Build history of the part. All positions in model axes, mm. A direction names the side the tool comes from. Coordinates: 2 decimals unless noted, no trailing zeros. Order: outer loops, then holes, each group sorted by start corner. A loop starts at its lowest first (then second) coordinate and runs counter-clockwise, first axis right, second up. Notation, with made-up numbers: M 7,62 L 28,62 A25 ccw 28,88 Z; hole C -17,85 d6. An arc over 180 degrees is marked long. Use a Markdown table: item, result. Add a question column.
from build123d import *

# Parameters (mm, degrees)
SKETCH1_W           = 124
SKETCH1_H           = 84
BOSS_EXTRUDE1_DEPTH = 25
SKETCH2_W           = 112
SKETCH2_H           = 73
CUT_EXTRUDE1_DEPTH  = 20
SKETCH4_W           = 2
SKETCH4_H           = 7
SKETCH4_H_2         = 36.5
CUT_EXTRUDE2_DEPTH  = 20
FILLET1_R           = 2.5
SKETCH5_W           = 119
SKETCH5_H           = 5
BOSS_EXTRUDE2_DEPTH = 10
SKETCH6_W           = 117
SKETCH6_H           = 4
BOSS_EXTRUDE3_DEPTH = 10
SKETCH7_R           = 2.5
CUT_EXTRUDE3_DEPTH  = 85.693565281


with BuildPart() as part:
    # Sketch1 → Boss-Extrude1 (new body)
    with BuildSketch(Plane(origin=(0, 0, 0), x_dir=(1, 0, 0), z_dir=(0, 1, 0))):
        Rectangle(SKETCH1_W, SKETCH1_H)
    extrude(amount=BOSS_EXTRUDE1_DEPTH)

    # Sketch2 → Cut-Extrude1 (cut)
    with BuildSketch(Plane(origin=(0, 25, 0), x_dir=(1, 0, 0), z_dir=(0, 1, 0))):
        with Locations((4, 0)):
            Rectangle(SKETCH2_W, SKETCH2_H)
    extrude(amount=-CUT_EXTRUDE1_DEPTH, mode=Mode.SUBTRACT)

    # Sketch4 → Cut-Extrude2 (cut)
    with BuildSketch(Plane(origin=(0, 25, 0), x_dir=(1, 0, 0), z_dir=(0, 1, 0))):
        with Locations((61, -24.5)):
            Rectangle(SKETCH4_W, SKETCH4_H)
        with Locations((61, 12.25)):
            Rectangle(SKETCH4_W, SKETCH4_H_2)
    extrude(amount=-CUT_EXTRUDE2_DEPTH, mode=Mode.SUBTRACT)

    # Fillet1
    fillet1_edges = [part.edges().sort_by_distance(p)[0] for p in [
        (62, 12.5, 42),
        (-62, 12.5, 42),
        (-62, 12.5, -42),
        (62, 12.5, -42),
    ]]
    fillet(fillet1_edges, radius=FILLET1_R)

    # Sketch5 → Boss-Extrude2 (add)
    with BuildSketch(Plane.XY.offset(42)):
        with Locations((0, 22.5)):
            Rectangle(SKETCH5_W, SKETCH5_H)
    extrude(amount=BOSS_EXTRUDE2_DEPTH)

    # Sketch6 → Boss-Extrude3 (add)
    with BuildSketch(Plane(origin=(0, 0, -42), x_dir=(-1, 0, 0), z_dir=(0, 0, -1))):
        with Locations((-1, 23)):
            Rectangle(SKETCH6_W, SKETCH6_H)
    extrude(amount=BOSS_EXTRUDE3_DEPTH)

    # Sketch7 → Cut-Extrude3 (cut, through all)
    with BuildSketch(Plane(origin=(0, 25, 0), x_dir=(1, 0, 0), z_dir=(0, 1, 0))):
        with Locations(Location((0, 47, 0), (0, 0, 270))):
            Circle(SKETCH7_R)
        with Locations(Location((0, -47, 0), (0, 0, 270))):
            Circle(SKETCH7_R)
    extrude(amount=-CUT_EXTRUDE3_DEPTH, mode=Mode.SUBTRACT)


solid = part.part
(1) Slice it at C-C on z = -47. Give the cut face in (x, y), and give its area (3 significant figures).
(2) Drop flat-ended pins along their axis: P1, Ø12.5, axis at x = -24, y = 14, coming from the -Z side; P2, Ø3, axis at y = 23, z = -47.5, coming from the -X side; P3, Ø1.5, axis at y = 21.5, z = 44.5, coming from the +X side. Give the stop position or say it passes through.
(3) Drill centre lines: line 1 along Z through (x, y) = (0.5, 15.75); line 2 along X through (y, z) = (9.25, 33); line 3 along X through (y, z) = (22.05, -47). Where is each one in solid material? Low to high. Write a range as from..to.
(4) Slice it at D-D on z = 33. Give the cut face in (x, y).
(5) Slice it at B-B on x = 0. Give the cut face in (y, z), and give its area (3 significant figures).
(6) Slice it at A-A on y = 13.75. Give the cut face in (x, z), and give its area (3 significant figures).
(7) Which spindle directions (+Z, -Z, +X, -X, +Y, -Y) get a long thin tool onto all of the face, cutting with end or side? Do faces 4 (the flat face through (-59.5, 22, 47)), 5 (the flat face through (-57.5, 23, -47)), 6 (the flat face through (2, 21, -45)), 7 (the flat face through (59.5, 22, 47)), 8 (the flat face through (60, 15, 14)). Say none if no direction does.
(8) Mould opens along X. For faces 1 (the flat face through (3, 15, -36.5)), 2 (the flat face through (-1, 10, -42)), 3 (the flat face through (-62, 12, 1)) say: released by +X, released by -X, zero draft, split by the parting line, or undercut.
Solutions:
| question | item | result |
|---|---|---|
| 1 | outline | M -57.5,21 L -2.5,21 L -2.5,25 L -57.5,25 Z; M 2.5,21 L 59.5,21 L 59.5,25 L 2.5,25 Z |
| 1 | area | 448 mm² |
| 2 | P1 | z = -42 |
| 2 | P2 | x = -57.5 |
| 2 | P3 | x = 59.5 |
| 3 | line 1 | -42..-36.5, 36.5..42 |
| 3 | line 2 | -62..-52, 60..62 |
| 3 | line 3 | -57.5..-2.5, 2.5..59.5 |
| 4 | outline | M -62,0 L 62,0 L 62,25 L 60,25 L 60,5 L -52,5 L -52,25 L -62,25 Z |
| 5 | outline | M 0,-42 L 21,-42 L 21,-44.5 L 25,-44.5 L 25,-36.5 L 5,-36.5 L 5,36.5 L 25,36.5 L 25,44.5 L 20,44.5 L 20,42 L 0,42 Z; M 20,49.5 L 25,49.5 L 25,52 L 20,52 Z; M 21,-52 L 25,-52 L 25,-49.5 L 21,-49.5 Z |
| 5 | area | 685 mm² |
| 6 | outline | M -62,-39.5 A2.5 ccw -59.5,-42 L 59.5,-42 A2.5 ccw 62,-39.5 L 62,-30.5 L 60,-30.5 L 60,-36.5 L -52,-36.5 L -52,36.5 L 60,36.5 L 60,28 L 62,28 L 62,39.5 A2.5 ccw 59.5,42 L -59.5,42 A2.5 ccw -62,39.5 Z; M 60,6 L 62,6 L 62,21 L 60,21 Z |
| 6 | area | 2,150 mm² |
| 7 | face 4 | +Z, -X, +Y, -Y |
| 7 | face 5 | -Z, -X, +Y, -Y |
| 7 | face 6 | -Z, +X, -X, -Y |
| 7 | face 7 | +Z, +X, +Y, -Y |
| 7 | face 8 | +Y |
| 8 | face 1 | undercut |
| 8 | face 2 | zero draft |
| 8 | face 3 | released by -X |
